Work out the finished part from the listing and answer in its coordinate system (mm). A direction names the side the tool comes from. Round coordinates to 2 decimals unless told otherwise and drop trailing zeros. Order: outer loops, then holes, each group sorted by start corner. A loop starts at its lowest first (then second) coordinate and runs counter-clockwise, first axis right, second up. Notation, with made-up numbers: M 19,66.25 L 71,66.25 A12 cw 71,77.25 Z; hole C 25.5,-40 d4. An arc over 180 degrees is marked long. Return JSON: item names as keys, results as strings.
from build123d import *

# Parameters (mm, degrees)
CROQUIS1_R              = 5.8
CROQUIS1_R_2            = 5
SALIENTE_EXTRUIR1_DEPTH = 0.8
CROQUIS1_3_R            = 5
CROQUIS1_3_R_2          = 2.5
SALIENTE_EXTRUIR2_DEPTH = 4
CHAFL_N1_SIZE           = 0.15


with BuildPart() as part:
    # Croquis1 → Saliente-Extruir1 (new body)
    with BuildSketch(Plane(origin=(0, 0, 0), x_dir=(1, 0, 0), z_dir=(0, 1, 0))):
        with Locations(Location((0, 0, 0), (0, 0, 270))):
            Circle(CROQUIS1_R)
        with Locations(Location((0, 0, 0), (0, 0, 270))):
            Circle(CROQUIS1_R_2, mode=Mode.SUBTRACT)
    extrude(amount=SALIENTE_EXTRUIR1_DEPTH)

    # Croquis1_3 → Saliente-Extruir2 (add)
    with BuildSketch(Plane(origin=(0, 0, 0), x_dir=(1, 0, 0), z_dir=(0, 1, 0))):
        with Locations(Location((0, 0, 0), (0, 0, 270))):
            Circle(CROQUIS1_3_R)
        with Locations(Location((0, 0, 0), (0, 0, 270))):
            Circle(CROQUIS1_3_R_2, mode=Mode.SUBTRACT)
    extrude(amount=SALIENTE_EXTRUIR2_DEPTH)

    # Chafl_n1
    chafl_n1_edges = [part.edges().sort_by_distance(p)[0] for p in [
        (0, 4, -2.5),
        (0, 4, -5),
        (0, 0, -2.5),
    ]]
    chamfer(chafl_n1_edges, length=CHAFL_N1_SIZE)


solid = part.part
Item 1: Each of these flat-tipped pins is pushed along its axis until it touches: pin 1 (2 mm diameter, centred on x = 4, y = 2.5, fed in from +Z); pin 2 (1 mm diameter, centred on x = 4, y = 3.5, fed in from +Z). Where does it stop, or does it pass through?
Output:
{"pin 1": "stops at z = 4", "pin 2": "stops at z = 3.57"}
Item 2: Consider line 1 along X through (y, z) = (2.5, 0); line 2 along Z through (x, y) = (-0.25, 3); line 3 along Y through (x, z) = (4.5, 3.25). Determine where each line is inside the solid, lowest interval first. Write a range as [from, to].
Output:
{"line 1": "x = [-5, -2.5], [2.5, 5]", "line 2": "z = [-4.99, -2.49], [2.49, 4.99]", "line 3": "y = [0, 0.8]"}
Item 3: The mould has two halves that part along X. Classify faces 3 (the cylindrical face through (0.255, 0.394, -5.794)), 4 (the cylindrical face through (-2.44, 1.97, -0.54)), 5 (the flat face through (3, 0, 0)): pulls with the +X half, pulls with the -X half, needs draft (parallel to the pull), parting line crosses it, or undercut.
Output:
{"face 3": "parting line crosses it", "face 4": "undercut", "face 5": "needs draft"}
Item 4: Find section C-C (y = 3.5). Determine the outline of the cut face in (x, z), plus the area to 3 significant figures.
Output:
{"outline": "C 0,0 d10; hole C 0,0 d5", "area": "58.9 mm^2"}
Item 5: Which of the six approach directions +Z, -Z, +X, -X, +Y, -Y give full straight-line access (tool end or side, diameter ignored) to faces 1 (the flat face through (-2, 4, 2)), 2 (the flat face through (5, 0.8, 2))?
Output:
{"face 1": "+Z, -Z, +X, -X, +Y", "face 2": "+Y"}
Item 6: Find section A-A (x = 0). Determine the outline of the cut face in (y, z), plus the area to 3 significant figures.
Output:
{"outline": "M 0,-5.8 L 0.8,-5.8 L 0.8,-5 L 3.85,-5 L 4,-4.85 L 4,-2.65 L 3.85,-2.5 L 0.15,-2.5 L 0,-2.65 Z; M 0,2.65 L 0.15,2.5 L 3.85,2.5 L 4,2.65 L 4,4.85 L 3.85,5 L 0.8,5 L 0.8,5.8 L 0,5.8 Z", "area": "21.2 mm^2"}
Item 7: Find section B-B (z = 0). Determine the outline of the cut face in (x, y), plus the area to 3 significant figures.
Output:
{"outline": "M -5.8,0 L -2.65,0 L -2.5,0.15 L -2.5,3.85 L -2.65,4 L -4.85,4 L -5,3.85 L -5,0.8 L -5.8,0.8 Z; M 2.5,0.15 L 2.65,0 L 5.8,0 L 5.8,0.8 L 5,0.8 L 5,3.85 L 4.85,4 L 2.65,4 L 2.5,3.85 Z", "area": "21.2 mm^2"}
